Can you work these out from the model? Positions are in its coordinate system, mm. A direction names the side the tool comes from. Give positions to 0.01 mm unless a question says otherwise; leave off trailing zeros. Order: outer loops, then holes, each group sorted by start corner. A loop starts at its lowest first (then second) coordinate and runs counter-clockwise, first axis right, second up. Notation, with made-up numbers: M -6.5,32 L 23.5,32 A15 ccw 23.5,46 Z; hole C 32.25,36.5 d10. An arc over 180 degrees is marked long. Answer as a JSON object with one key per item and string values.
```python
from build123d import *

# Parameters (mm, degrees)
ESQUISSE1_R          = 7
BASE_EXTRUSION_DEPTH = 5
CONG_1_R             = 3
ESQUISSE2_R          = 4
BOSS_EXTRU_2_DEPTH   = 4


with BuildPart() as part:
    # Esquisse1 → Base-Extrusion (new body)
    with BuildSketch(Plane.XY):
        Circle(ESQUISSE1_R)
    extrude(amount=BASE_EXTRUSION_DEPTH)

    # Congé1
    cong_1_edges = [part.edges().sort_by_distance(p)[0] for p in [
        (-7, 0, 0),
    ]]
    fillet(cong_1_edges, radius=CONG_1_R)

    # Esquisse2 → Boss.-Extru.2 (add)
    with BuildSketch(Plane.XY.offset(5)):
        Circle(ESQUISSE2_R)
    extrude(amount=BOSS_EXTRU_2_DEPTH)


solid = part.part
```
1) I want a section at A-A on y = 0. Write out the boundary of the cut face in (x, z), and give its area (3 significant figures).
Results found:
{"outline": "M -7,3 A3 ccw -4,0 L 4,0 A3 ccw 7,3 L 7,5 L 4,5 L 4,9 L -4,9 L -4,5 L -7,5 Z", "area": "98.1 mm²"}
2) I'm going to push flat-ended pins straight in: pin 1 Ø4 at (x, z) = (-4, 3) entering from +Y; pin 2 Ø2 at (x, z) = (0, 1.5) entering from +Y; pin 3 Ø1 at (x, y) = (-3, 5.5) entering from +Z. Where does each tip first touch, or does it pass through?
Results found:
{"pin 1": "stops at y = 6.71", "pin 2": "stops at y = 6.96", "pin 3": "stops at z = 5"}
3) I need wall thicknesses on L1, parallel to Y at x = 0.25, z = 4.25; L2, parallel to X at y = -5, z = 3.5; L3, parallel to Y at x = -5.25, z = 4. Which ranges of each line are inside material? Lowest first, please.
Results found:
{"L1": "y = -7 to 7", "L2": "x = -4.9 to 4.9", "L3": "y = -4.63 to 4.63"}
4) For faces 1 (the face through (0, 0, 9)), 2 (the face through (-0.867, -3.905, 6.972)), which set-ups out of +Z, -Z, +X, -X, +Y, -Y let a thin tool reach every point of the face, with its end or its side?
Results found:
{"face 1": "+Z, +X, -X, +Y, -Y", "face 2": "+Z"}
5) I want a section at C-C on z = 8.75. Write out the boundary of the cut face in (x, y).
Results found:
{"outline": "C 0,0 d8"}
